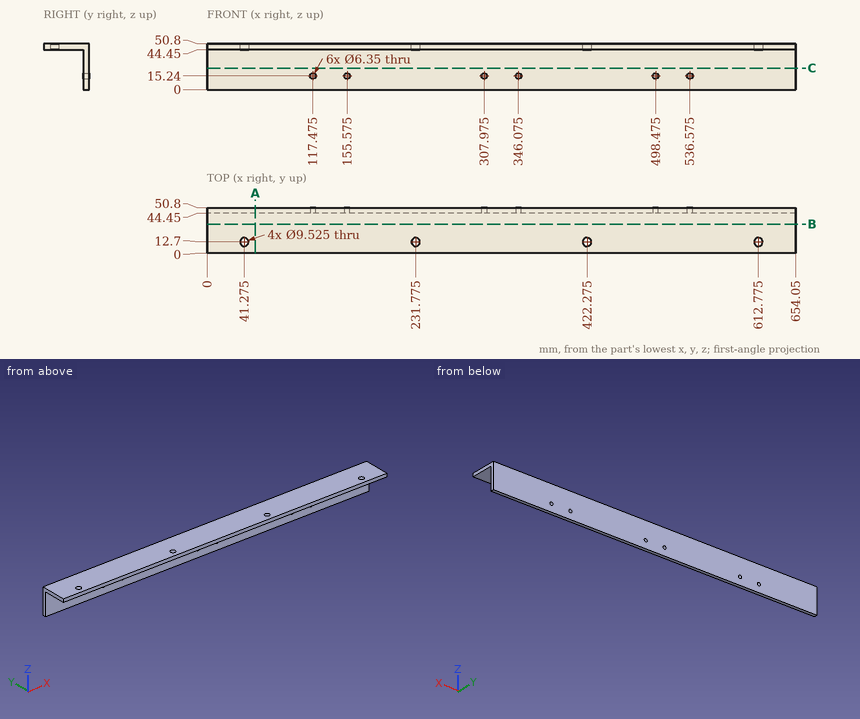
The figure shows three views and two pictorial views of one solid part (mm, origin at its lowest corner). Answer the questions. Give positions to 0.01 mm unless a question says otherwise; leave off trailing zeros. Order: outer loops, then holes, each group sorted by start corner. A loop starts at its lowest first (then second) coordinate and runs counter-clockwise, first axis right, second up. Notation, with made-up numbers: (33, 71) -> (71, 71) arc R24 cw to (71, 91) -> close; hole circle Ø9 at (21.5, 2.5). An arc over 180 degrees is marked (long way). Answer as CSV lines item,"result". Start each with the question number.
(1) Section A-A, the plane x = 53.5 is taken. Write down the section's boundary in (y, z), plus the area to 3 significant figures.
(2) Section B-B, the plane y = 32.5 is taken. Write down the section's boundary in (x, z), plus the area to 3 significant figures.
(3) Consider line 1 along X through (y, z) = (12, 48); line 2 along Y through (x, z) = (33.5, 10.5). Determine where each line is inside the solid, lowest interval first.
(4) Each of these flat-tipped pins is pushed along its axis until it touches: pin 1 Ø11 at (x, y) = (231.775, 12.7) entering from -Z; pin 2 Ø4 at (x, z) = (536.575, 15.24) entering from -Y; pin 3 Ø10 at (x, z) = (498.475, 15.24) entering from -Y. Where does it stop, or does it pass through?
Entries:
1,outline,"(0, 44.45) -> (44.45, 44.45) -> (44.45, 0) -> (50.8, 0) -> (50.8, 50.8) -> (0, 50.8) -> close"
1,area,"605 mm²"
2,outline,"(0, 44.45) -> (654.05, 44.45) -> (654.05, 50.8) -> (0, 50.8) -> close"
2,area,"4,150 mm²"
3,line 1,"0 to 36.56, 45.99 to 227.06, 236.49 to 417.56, 426.99 to 608.06, 617.49 to 654.05"
3,line 2,"44.45 to 50.8"
4,pin 1,"z = 44.45"
4,pin 2,"through"
4,pin 3,"y = 44.45"
